Part print with two shaded views. Sizes in mm from the minimum x, y, z corner. Round coordinates to 2 decimals unless told otherwise and drop trailing zeros. Order: outer loops, then holes, each group sorted by start corner. A loop starts at its lowest first (then second) coordinate and runs counter-clockwise, first axis right, second up. Notation, with made-up numbers: M 20.5,49.5 L 63.5,49.5 A14 cw 63.5,55.5 Z; hole C 32,-30.5 d2. An arc over 180 degrees is marked long. Return JSON: item names as keys, results as strings. Group by question number.
Item 1: Pin check, flat tips, straight feed: pin 1 Ø4 at (x, y) = (4.5, 3) entering from -Z; pin 2 Ø1.5 at (y, z) = (5.5, 2.5) entering from -X; pin 3 Ø4 at (y, z) = (11, 2.5) entering from -X (1 decimal). Stop position of each tip, or through.
Item 2: Pull direction Y, two halves, no side cores. Call the marked faces 1, 2 and 3: pulls with the +Y half, pulls with the -Y half, needs draft (parallel to the pull), parting line crosses it, or undercut.
Item 3: Probe line 1 along Y through (x, z) = (9, 4) (1 decimal); line 2 along X through (y, z) = (6.5, 6.5); line 3 along X through (y, z) = (6.75, 7.5). List the from-to ranges inside material, lowest first.
Item 4: Slice it at A-A on z = 2. Write the cut outline in (x, y) (1 decimal), then the cut area to 3 significant figures.
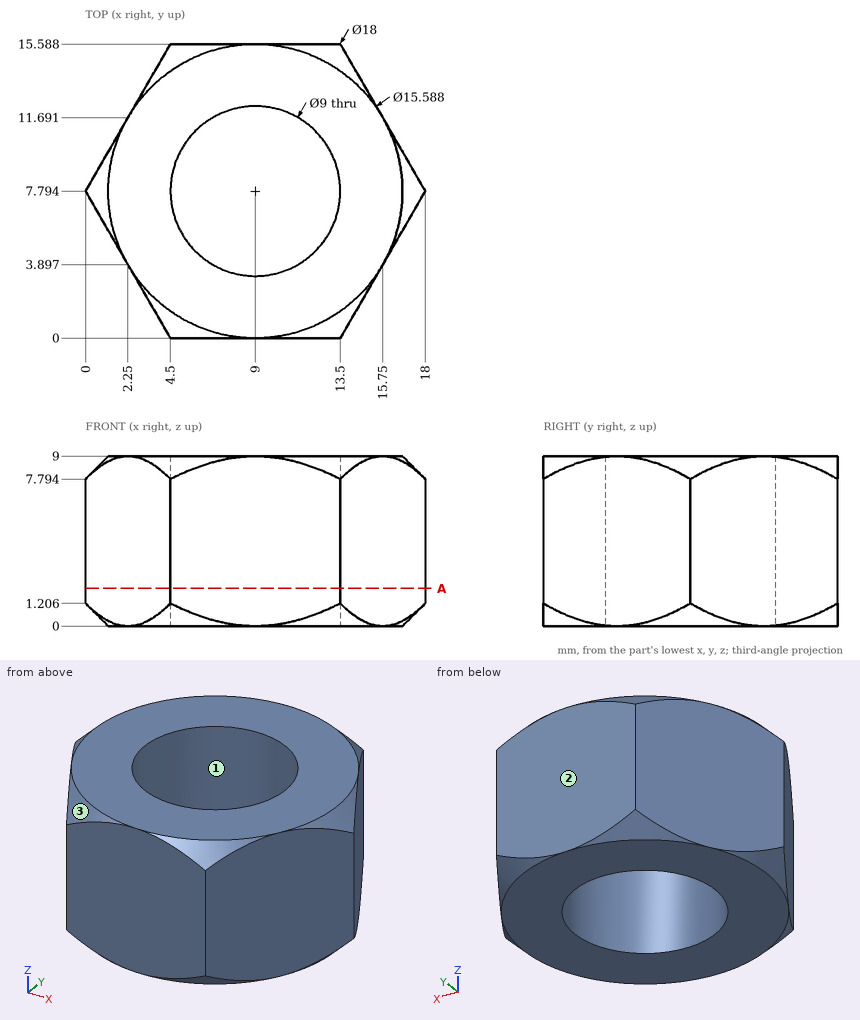
Output values:
{
 "1": {"pin 1": "z = 0", "pin 2": "x = 0.89", "pin 3": "x = 0.7"},
 "2": {"face 1": "undercut", "face 2": "pulls with the +Y half", "face 3": "pulls with the -Y half"},
 "3": {"line 1": "0 to 3.3, 12.3 to 15.6", "line 2": "0.75 to 4.69, 13.31 to 17.25", "line 3": "0.6 to 4.62, 13.38 to 17.4"},
 "4": {"outline": "M 0,7.8 L 4.5,0 L 13.5,0 L 18,7.8 L 13.5,15.6 L 4.5,15.6 Z; hole C 9,7.8 d9", "area": "147 mm²"}
}
